Model file for the job. Use its own axes, mm. Face numbers are marked on the shaded views. A direction names the side the tool comes from. Coordinates: 2 decimals unless noted, no trailing zeros. Loops run counter-clockwise (first coordinate to the right, second up) from the corner with the lowest first, then second, coordinate; pieces in that order, holes last.
Autodesk Inventor part; units mm, degrees
ref_plane "YZ Plane" through (0, 0, 0) normal (1, 0, 0) x (0, 1, 0)
ref_plane "XZ Plane" through (0, 0, 0) normal (0, 1, 0) x (-1, 0, 0)
ref_plane "XY Plane" through (0, 0, 0) normal (0, 0, 1) x (1, 0, 0)
sketch "Sketch1" plane through (0, 0, 0) normal (0, 1, 0) x (-1, 0, 0)
  circle A0 centre (0, 0) radius 12
  dimension "d0" = 24
extrude "Extrusion1" add sketch "Sketch1" along normal blind 30.5
sketch "Sketch2" plane through (0, 30.5, 0) normal (0, 1, 0) x (1, 0, 0)
  circle A0 centre (0, 0) radius 12
  circle A1 centre (0, 0) radius 12.2
  dimension "d3" = 24.4
extrude "Extrusion2" add sketch "Sketch2" along normal blind 24 contours A0 | A1
sketch "Sketch3" plane through (0, 54.5, 0) normal (0, 1, 0) x (1, 0, 0)
  circle A0 centre (0, 0) radius 6
  dimension "d6" = 12
extrude "Extrusion3" add sketch "Sketch3" along normal blind 3.25
sketch "Sketch4" plane through (0, 54.5, 0) normal (0, 1, 0) x (1, 0, 0)
  circle A0 centre (0, 0) radius 6
  circle A1 centre (0, 0) radius 12.2
  line L0 (0, 0) -> (-7.5, 0)
  circle A2 centre (-7.5, 0) radius 3
  circle A3 centre (0, -7.5) radius 3
  circle A4 centre (7.5, 0) radius 3
  circle A5 centre (0, 7.5) radius 3
  point P0 (-5.55, 2.2798)
  point P1 (-5.55, -2.2798)
  point P2 (2.2798, 5.55)
  point P3 (-2.2798, 5.55)
  point P4 (5.55, -2.2798)
  point P5 (5.55, 2.2798)
  point P6 (-2.2798, -5.55)
  point P7 (2.2798, -5.55)
  dimension "d9" = 7.5
  dimension "d10" = 6
  dimension "d13" = 360
extrude "Extrusion4" add sketch "Sketch4" along normal blind 3.25 contours A0 A4 | A0 A5 | A3 A0 | A0 A2 picked at (7.2585, 0.8906) picked at (-1.2671, 6.9374) picked at (-1.2671, -6.9374)
sketch "Sketch5" plane through (0, 57.75, 0) normal (0, 1, 0) x (1, 0, 0)
  arc A0 (5.55, 2.2798) -> (2.2798, 5.55) centre (0, 0) ccw
  arc A1 (2.2798, 5.55) -> (-2.2798, 5.55) centre (0, 7.5) ccw
  arc A2 (-2.2798, 5.55) -> (-5.55, 2.2798) centre (0, 0) ccw
  arc A3 (-5.55, 2.2798) -> (-5.55, -2.2798) centre (-7.5, 0) ccw
  arc A4 (-5.55, -2.2798) -> (-2.2798, -5.55) centre (0, 0) ccw
  arc A5 (-2.2798, -5.55) -> (2.2798, -5.55) centre (0, -7.5) ccw
  arc A6 (2.2798, -5.55) -> (5.55, -2.2798) centre (0, 0) ccw
  arc A7 (5.55, -2.2798) -> (5.55, 2.2798) centre (7.5, 0) ccw
hole "Hole1" at (-7.5, 57.75, 0) at (0, 57.75, 7.5) at (7.5, 57.75, 0) at (0, 57.75, -7.5) direction (0, -1, 0) diameter 3 depth 5 tip angle 118
sketch "Sketch6" plane through (0, 57.75, 0) normal (0, 1, 0) x (1, 0, 0)
  circle A0 centre (0, 0) radius 5
  dimension "d24" = 10
extrude "Extrusion5" add sketch "Sketch6" along normal blind 2.5
sketch "Sketch7" plane through (0, 60.25, 0) normal (0, 1, 0) x (1, 0, 0)
  circle A0 centre (0, 0) radius 2.25
  dimension "d27" = 4.5
extrude "Extrusion6" add sketch "Sketch7" along normal blind 14.5
sketch "Sketch8" plane through (0, 0, 0) normal (0, -1, 0) x (1, 0, 0)
  circle A0 centre (0, 0) radius 4.125
  dimension "d30" = 8.25
extrude "Extrusion7" add sketch "Sketch8" along normal blind 2
sketch "Sketch9" plane through (0, -2, 0) normal (0, -1, 0) x (1, 0, 0)
  circle A0 centre (0, 0) radius 4.125
  circle A1 centre (0, 0) radius 1
  dimension "d33" = 2
extrude "Extrusion8" add sketch "Sketch9" along normal blind 0.5 contours A1
sketch "Sketch10" plane through (0, 0, 0) normal (0, -1, 0) x (1, 0, 0)
  circle A0 centre (0, 0) radius 4.125
  circle A1 centre (0, 0) radius 12
  line L0 (0, 0) -> (0, -6.5)
  line L1 (0, 0) -> (0, 6.5)
  circle A2 centre (0, 6.5) radius 1
  circle A3 centre (0, -6.5) radius 1
  dimension "d36" = 6.5
  dimension "d37" = 6.5
  dimension "d38" = 2
  dimension "d39" = 2
extrude "Extrusion9" cut sketch "Sketch10" against normal blind 0.5 contours A3 | A2
sketch "Sketch11" plane through (0, 0, 0) normal (0, -1, 0) x (1, 0, 0)
  circle A0 centre (0, -6.5) radius 1
  circle A1 centre (0, 6.5) radius 1
  circle A2 centre (0, 0) radius 4.125
  circle A3 centre (0, 0) radius 12
  line L0 (0, 0) -> (0, -10.15)
  line L1 (0, 0) -> (0, 10.15)
  circle A4 centre (0, 10.15) radius 1.4
  circle A5 centre (0, -10.15) radius 1.4
  arc A6 (2.2798, 5.55) -> (-2.2798, 5.55) centre (0, 7.5) ccw
  line L2 (1.4, 10.1533) -> (-1.4, 10.1533)
  line L3 (-1.4, 10.1533) -> (-1.4, 13.1533)
  line L4 (-1.4, 13.1533) -> (1.4, 13.1533)
  line L5 (1.4, 13.1533) -> (1.4, 10.1533)
  arc A7 (-2.2798, -5.55) -> (2.2798, -5.55) centre (0, -7.5) ccw
  line L6 (1.4, -10.1533) -> (-1.4, -10.1533)
  line L7 (-1.4, -10.1533) -> (-1.4, -13.1533)
  line L8 (-1.4, -13.1533) -> (1.4, -13.1533)
  line L9 (1.4, -13.1533) -> (1.4, -10.1533)
  point P0 (-1.4, -10.1533)
  point P1 (-1.4, -11.9181)
  point P2 (1.4, -11.9181)
  point P3 (1.4, 11.9181)
  point P4 (-1.4, 11.9181)
  point P5 (-1.4, 10.1533)
  dimension "d44" = 2.8
  dimension "d45" = 2.8
  dimension "d42" = 10.15
  dimension "d43" = 10.15
  dimension "d46" = 2.8
  dimension "d47" = 3
  dimension "d48" = 2.8
  dimension "d49" = 3
extrude "Extrusion10" cut sketch "Sketch11" against normal blind 1 contours A5 L6 | A7 A5 | L6 A7 | A5 L9 A3 L7 | A3 L5 A4 L3 | A4 L2 | A4 A6 | A6 L2
sketch "Sketch12" plane through (0, 0, 0) normal (0, -1, 0) x (1, 0, 0)
  line L0 (1.4, -10.1533) -> (1.4, -11.9181)
  arc A0 (1.4, -11.9181) -> (1.4, 11.9181) centre (0, 0) ccw
  line L1 (1.4, 11.9181) -> (1.4, 10.1533)
  arc A1 (-1.4, 10.1533) -> (1.4, 10.1533) centre (0, 10.15) ccw
  line L2 (-1.4, 10.1533) -> (-1.4, 11.9181)
  arc A2 (-1.4, 11.9181) -> (-1.4, -11.9181) centre (0, 0) ccw
  line L3 (-1.4, -11.9181) -> (-1.4, -10.1533)
  arc A3 (1.4, -10.1533) -> (-1.4, -10.1533) centre (0, -10.15) ccw
  circle A4 centre (0, -6.5) radius 1
  circle A5 centre (0, 6.5) radius 1
  circle A6 centre (0, 0) radius 4.125
  circle A7 centre (0, 0) radius 5.25
  circle A8 centre (0, 0) radius 7.5
  line L4 (0, 0) -> (7.5, 0)
  line L5 (0, 0) -> (3.75, -6.4952)
  line L6 (0, 0) -> (3.75, 6.4952)
  point P0 (2.625, 4.5466)
  point P1 (2.625, -4.5466)
  dimension "d52" = 10.5
  dimension "d53" = 15
  dimension "d54" = 60
  dimension "d55" = 60
extrude "Extrusion11" cut sketch "Sketch12" against normal blind 0.5 contours L5 A7 L4 A8 | A8 L4 A7 L6
fillet "Fillet1" radius 1 4 edges at (3.75, 0.25, 6.4952) (2.625, 0.25, 4.5466) (2.625, 0.25, -4.5466) (3.75, 0.25, -6.4952)
pattern_circular "Circular Pattern1" count 2 over 360 about axis through (0, 0, 0) along (0, -1, 0) of "Extrusion11", "Fillet1"
properties part number "motor_2"
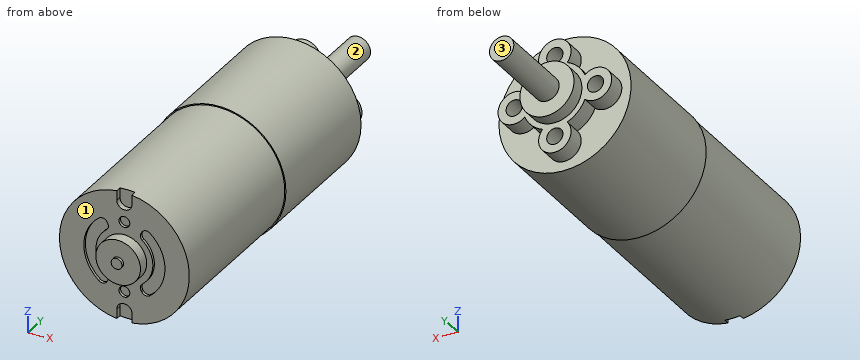
Q1. Which spindle directions (+Z, -Z, +X, -X, +Y, -Y) get a long thin tool onto all of the face, cutting with end or side? Do the marked faces 1, 2 and 3. Say none if no direction does.
Answers:
face 1: -Y
face 2: +Y
face 3: +Z, -Z, +X, -X, +Y
Q2. Slice it at B-B (y = 19). List the corners of the cut face in (x, z).
Answers:
outline: circle Ø24 at (0, 0)
Q3. Drill centre lines: line 1 (Z direction, x = 0, y = 56.15); line 2 (Z direction, x = 0, y = 0.35). Where is each one in solid material? Low to high.
Answers:
line 1: z = -10.5 to -9, -6 to 6, 9 to 10.5
line 2: z = -8.75 to -7.5, -5.5 to 5.5, 7.5 to 8.75
Q4. Flat gauge pins, fed straight in: P1, Ø12, axis at y = 26, z = 7, coming from the -X side; P2, Ø2.5, axis at x = 0, z = 6.5, coming from the +Y side; P3, Ø1.4, axis at x = -5.5, z = 0, coming from the -Y side. Where does each tip first touch, or does it go through?
Answers:
P1: stops at x = -11.96
P2: stops at y = 57.75
P3: stops at y = 0
Q5. Slice it at A-A (y = 39.5). List the corners of the cut face in (x, z).
Answers:
outline: circle Ø24.4 at (0, 0)
